The listing builds one solid part. Answer for the finished solid, in the listing's coordinates (mm). A direction names the side the tool comes from. Round coordinates to 2 decimals unless told otherwise and drop trailing zeros. Loops run counter-clockwise (first coordinate to the right, second up) from the corner with the lowest first, then second, coordinate; pieces in that order, holes last. Notation, with made-up numbers: (50, 78.25) -> (95, 78.25) arc R13 cw to (95, 102.25) -> close; hole circle Ø5 at (55, 49). An arc over 180 degrees is marked (long way). Use a Markdown table: item, result. Add a question column.
Q1. Consider line 1 (X direction, y = 17, z = 20); line 2 (Y direction, x = 20, z = 18.5); line 3 (X direction, y = -3.25, z = -10). Determine where each line is inside the solid, lowest interval first.
Q2. Section A-A on x = 20 is taken. Give the vertices of the cut face in (y, z), then the cut area to 3 significant figures.
Q3. Section C-C on z = 12 is taken. Give the vertices of the cut face in (x, y), then the cut area to 3 significant figures.
Q4. Section B-B on z = 18 is taken. Give the vertices of the cut face in (x, y), then the cut area to 3 significant figures.
Q5. Which of the six approach directions +Z, -Z, +X, -X, +Y, -Y give full straight-line access (tool end or side, diameter ignored) to faces 1 (the flat face through (0, 17.75, 19)), 2 (the flat face through (-11.75, 11, 0)), 3 (the flat face through (16, 0, 12)), 4 (the flat face through (0, -4, 20))?
Q6. For a pull along Z with two mould halves and no side action, classify faces 5 (the flat face through (0, 35, 17)), 6 (the flat face through (16, 0, -10)), 7 (the flat face through (12.5, 16, 19)), 8 (the cylindrical face through (18.233, -2.465, -9.74)) as released by +Z, released by -Z, zero draft, split by the parting line, or undercut.
Q7. Section D-D on x = -16.25 is taken. Give the vertices of the cut face in (y, z), then the cut area to 3 significant figures.
Q8. Given pin 1 Ø3 at (x, z) = (14.5, 15) entering from +Y; pin 2 Ø4 at (x, y) = (-20, 17) entering from -Z; pin 3 Ø0.8 at (x, z) = (5, 19.5) entering from -Y, each flat-ended and moving along its own axis, determine where each tip first touches the part or whether it passes through.
from build123d import *

# Parameters (mm, degrees)
SKETCH1_W                      = 46.5
SKETCH1_H                      = 34
BOSS_EXTRUDE1_DEPTH            = 13.75
SKETCH2_W                      = 46.5
SKETCH2_H                      = 42.25
BOSS_EXTRUDE2_DEPTH            = 2
SKETCH4_W                      = 35
SKETCH4_H                      = 12
CUT_EXTRUDE2_DEPTH             = 5
SKETCH6_W                      = 46.5
SKETCH6_H                      = 36
SKETCH6_R                      = 2
BOSS_EXTRUDE3_DEPTH            = 5
SKETCH8_W                      = 46.5
SKETCH8_H                      = 2.5
BOSS_EXTRUDE4_DEPTH            = 46.25
CUT_EXTRUDE1_REACH             = 62.18
SKETCH3_R                      = 1.25
SKETCH3_W                      = 25
SKETCH3_H                      = 10
CUT_EXTRUDE1_DIRECTION_2_DEPTH = 51
SKETCH7_W                      = 25
SKETCH7_H                      = 4
CUT_EXTRUDE3_DEPTH             = 10


with BuildPart() as part:
    # Sketch1 → Boss-Extrude1 (new body)
    with BuildSketch(Plane(origin=(0, 0, 0), x_dir=(1, 0, 0), z_dir=(0, 1, 0))):
        Rectangle(SKETCH1_W, SKETCH1_H)
    extrude(amount=BOSS_EXTRUDE1_DEPTH)

    # Sketch2 → Boss-Extrude2 (add)
    with BuildSketch(Plane.XY.offset(17)):
        with Locations((0, 21.125)):
            Rectangle(SKETCH2_W, SKETCH2_H)
    extrude(amount=BOSS_EXTRUDE2_DEPTH)

    # Sketch4 → Cut-Extrude2 (cut)
    with BuildSketch(Plane(origin=(0, 13.75, 0), x_dir=(1, 0, 0), z_dir=(0, 1, 0))):
        with Locations((5.75, 0)):
            Rectangle(SKETCH4_W, SKETCH4_H)
    extrude(amount=-CUT_EXTRUDE2_DEPTH, mode=Mode.SUBTRACT)

    # Sketch6 → Boss-Extrude3 (add)
    with BuildSketch(Plane.XZ):
        with Locations((0, 1)):
            Rectangle(SKETCH6_W, SKETCH6_H)
        with Locations(Location((16.25, -10, 0), (0, 0, 270))):
            Circle(SKETCH6_R, mode=Mode.SUBTRACT)
        with Locations(Location((-16.25, -10, 0), (0, 0, 270))):
            Circle(SKETCH6_R, mode=Mode.SUBTRACT)
        with Locations(Location((-16.25, 12, 0), (0, 0, 270))):
            Circle(SKETCH6_R, mode=Mode.SUBTRACT)
        with Locations(Location((16.25, 12, 0), (0, 0, 270))):
            Circle(SKETCH6_R, mode=Mode.SUBTRACT)
    extrude(amount=BOSS_EXTRUDE3_DEPTH)

    # Sketch8 → Boss-Extrude4 (add)
    with BuildSketch(Plane(origin=(0, -4, 0), x_dir=(-1, 0, 0), z_dir=(0, -1, 0))):
        with Locations((0, -20.25)):
            Rectangle(SKETCH8_W, SKETCH8_H)
    extrude(amount=-BOSS_EXTRUDE4_DEPTH)

    # Sketch3 → Cut-Extrude1 (cut, up to next)
    with BuildSketch(Plane.XY.offset(19), mode=Mode.PRIVATE) as cut_extrude1_sk1:
        with Locations(Location((-20, 39, 0), (0, 0, 180))):
            Circle(SKETCH3_R)
    cut_extrude1_tool1 = extrude(cut_extrude1_sk1.sketch, amount=-CUT_EXTRUDE1_REACH, mode=Mode.PRIVATE) & part.part
    # Sketch3 → Cut-Extrude1 (cut, up to next)
    with BuildSketch(Plane.XY.offset(19), mode=Mode.PRIVATE) as cut_extrude1_sk2:
        with Locations(Location((20, 39, 0), (0, 0, 180))):
            Circle(SKETCH3_R)
    cut_extrude1_tool2 = extrude(cut_extrude1_sk2.sketch, amount=-CUT_EXTRUDE1_REACH, mode=Mode.PRIVATE) & part.part
    # Sketch3 → Cut-Extrude1 (cut, up to next)
    with BuildSketch(Plane.XY.offset(19), mode=Mode.PRIVATE) as cut_extrude1_sk3:
        with Locations(Location((20, 17, 0), (0, 0, 180))):
            Circle(SKETCH3_R)
    cut_extrude1_tool3 = extrude(cut_extrude1_sk3.sketch, amount=-CUT_EXTRUDE1_REACH, mode=Mode.PRIVATE) & part.part
    # Sketch3 → Cut-Extrude1 (cut, up to next)
    with BuildSketch(Plane.XY.offset(19), mode=Mode.PRIVATE) as cut_extrude1_sk4:
        with Locations(Location((-20, 17, 0), (0, 0, 180))):
            Circle(SKETCH3_R)
    cut_extrude1_tool4 = extrude(cut_extrude1_sk4.sketch, amount=-CUT_EXTRUDE1_REACH, mode=Mode.PRIVATE) & part.part
    # Sketch3 → Cut-Extrude1 (cut, up to next)
    with BuildSketch(Plane.XY.offset(19), mode=Mode.PRIVATE) as cut_extrude1_sk5:
        with Locations((0, 28)):
            Rectangle(SKETCH3_W, SKETCH3_H)
    cut_extrude1_tool5 = extrude(cut_extrude1_sk5.sketch, amount=-CUT_EXTRUDE1_REACH, mode=Mode.PRIVATE) & part.part
    add(cut_extrude1_tool1.solids().sort_by_distance((-20, 39, 19))[0], mode=Mode.SUBTRACT)
    add(cut_extrude1_tool2.solids().sort_by_distance((20, 39, 19))[0], mode=Mode.SUBTRACT)
    add(cut_extrude1_tool3.solids().sort_by_distance((20, 17, 19))[0], mode=Mode.SUBTRACT)
    add(cut_extrude1_tool4.solids().sort_by_distance((-20, 17, 19))[0], mode=Mode.SUBTRACT)
    add(cut_extrude1_tool5.solids().sort_by_distance((0, 28, 19))[0], mode=Mode.SUBTRACT)

    # Sketch3 → Cut-Extrude1 direction 2 (cut)
    with BuildSketch(Plane.XY.offset(19)):
        with Locations(Location((-20, 39, 0), (0, 0, 180))):
            Circle(SKETCH3_R)
        with Locations(Location((20, 39, 0), (0, 0, 180))):
            Circle(SKETCH3_R)
        with Locations(Location((20, 17, 0), (0, 0, 180))):
            Circle(SKETCH3_R)
        with Locations(Location((-20, 17, 0), (0, 0, 180))):
            Circle(SKETCH3_R)
        with Locations((0, 28)):
            Rectangle(SKETCH3_W, SKETCH3_H)
    extrude(amount=CUT_EXTRUDE1_DIRECTION_2_DEPTH, mode=Mode.SUBTRACT)

    # Sketch7 → Cut-Extrude3 (cut)
    with BuildSketch(Plane(origin=(0, 0, 17), x_dir=(-1, 0, 0), z_dir=(0, 0, -1))):
        with Locations((0, 15.75)):
            Rectangle(SKETCH7_W, SKETCH7_H)
        with Locations((0, 40.25)):
            Rectangle(SKETCH7_W, SKETCH7_H)
    extrude(amount=-CUT_EXTRUDE3_DEPTH, mode=Mode.SUBTRACT)


solid = part.part
Checked values:
| question | item | result |
|---|---|---|
| 1 | line 1 | x = -23.25 to -21.25, -18.75 to -12.5, 12.5 to 18.75, 21.25 to 23.25 |
| 1 | line 2 | y = -5 to 15.75, 18.25 to 37.75, 40.25 to 42.25 |
| 1 | line 3 | x = -23.25 to -18.25, -14.25 to 14.25, 18.25 to 23.25 |
| 2 | outline | (-5, -17) -> (13.75, -17) -> (13.75, -6) -> (8.75, -6) -> (8.75, 6) -> (13.75, 6) -> (13.75, 17) -> (15.75, 17) -> (15.75, 21.5) -> (-4, 21.5) -> (-4, 19) -> (-5, 19) -> close; (18.25, 17) -> (37.75, 17) -> (37.75, 21.5) -> (18.25, 21.5) -> close; (40.25, 17) -> (42.25, 17) -> (42.25, 21.5) -> (40.25, 21.5) -> close |
| 2 | area | 765 mm2 |
| 3 | outline | (-23.25, -5) -> (-18.25, -5) -> (-18.25, 0) -> (-14.25, 0) -> (-14.25, -5) -> (14.25, -5) -> (14.25, 0) -> (18.25, 0) -> (18.25, -5) -> (23.25, -5) -> (23.25, 13.75) -> (-23.25, 13.75) -> close |
| 3 | area | 832 mm2 |
| 4 | outline | (-23.25, -5) -> (23.25, -5) -> (23.25, 42.25) -> (12.5, 42.25) -> (12.5, 38.25) -> (-12.5, 38.25) -> (-12.5, 42.25) -> (-23.25, 42.25) -> close; hole circle Ø2.5 at (-20, 17); hole circle Ø2.5 at (-20, 39); hole (-12.5, 13.75) -> (12.5, 13.75) -> (12.5, 17.75) -> (-12.5, 17.75) -> close; hole (-12.5, 23) -> (12.5, 23) -> (12.5, 33) -> (-12.5, 33) -> close; hole circle Ø2.5 at (20, 17); hole circle Ø2.5 at (20, 39) |
| 4 | area | 1,730 mm2 |
| 5 | face 1 | +Z, -Z |
| 5 | face 2 | +X, +Y |
| 5 | face 3 | -Y |
| 5 | face 4 | +Z, +X, -X, -Y |
| 6 | face 5 | released by -Z |
| 6 | face 6 | undercut |
| 6 | face 7 | zero draft |
| 6 | face 8 | undercut |
| 7 | outline | (-5, -17) -> (13.75, -17) -> (13.75, 17) -> (42.25, 17) -> (42.25, 21.5) -> (-4, 21.5) -> (-4, 19) -> (-5, 19) -> (-5, 14) -> (0, 14) -> (0, 10) -> (-5, 10) -> (-5, -8) -> (0, -8) -> (0, -12) -> (-5, -12) -> close |
| 7 | area | 808 mm2 |
| 8 | pin 1 | stops at y = 13.75 |
| 8 | pin 2 | stops at z = 17 |
| 8 | pin 3 | stops at y = -4 |
